Geometry: final body of the model. Coordinates: model frame, mm. Round coordinates to 2 decimals unless told otherwise and drop trailing zeros. Write each loop counter-clockwise with the first axis right and the second up, starting at its lowest first coordinate (ties: lowest second). Pieces come first, ordered by that corner, then holes. Notation, with made-up numbers: M 57.25,-6 L 92.25,-6 A11 cw 92.25,0 Z; hole C 11.5,38.25 d7. An arc over 180 degrees is marked long. Answer as CSV lines item,"result". Start each with the question number.
Q1. Section query B-B on y = -1.5. Output: boundary loops of the cut face in (x, z), and give its area (3 significant figures).
Q2. Section query C-C on z = -825. Output: boundary loops of the cut face in (x, y).
Q3. Ray query, probe 1 along Z at (x, y) = (418, 36); probe 2 along X at (y, z) = (-106, -161). Return the intervals inside material, ascending.
Q4. Section query A-A on x = -86. Output: boundary loops of the cut face in (y, z), and give its area (3 significant figures).
```python
from build123d import *

# Parameters (mm, degrees)
F0_W     = 412.1005833149
F0_H     = 230.7337969542
F1_DEPTH = 15
F2_R     = 6.4013337275
F3_DEPTH = 1000
F4_DEPTH = 1000
F5_DEPTH = 134.62


with BuildPart() as f1:
    # F0 (on Top) → F1 (new body)
    with BuildSketch(Plane.XY):
        Rectangle(F0_W, F0_H)
    extrude(amount=F1_DEPTH)

    # F2 (on face) → F3 (join)
    with BuildSketch(Plane(origin=(0, 0, 0), x_dir=(1, 0, 0), z_dir=(0, 0, -1))):
        with Locations((-190.1699453592, 101.8757298589)):
            Circle(F2_R)
    extrude(amount=F3_DEPTH)

    # F4 (add): a face of the model
    f4_faces = [f1.faces().sort_by_distance(p)[0] for p in [
        (206.0502916574, 0, 7.5),
    ]]
    extrude(f4_faces, amount=F4_DEPTH)

    # F5 (add): a face of the model
    f5_faces = [f1.faces().sort_by_distance(p)[0] for p in [
        (500, -115.3668984771, 7.5),
    ]]
    extrude(f5_faces, amount=F5_DEPTH)


solid = f1.part
```
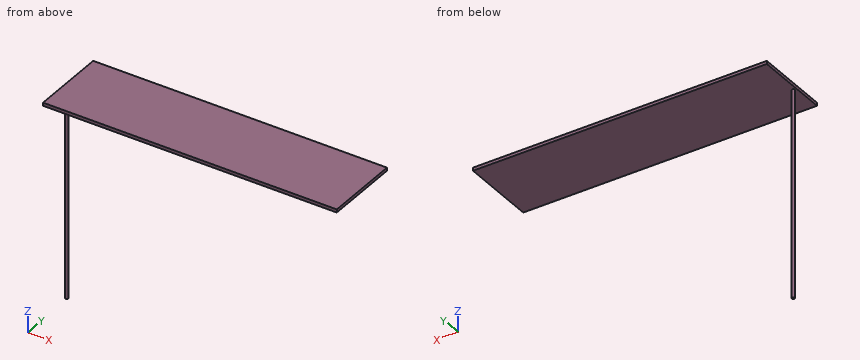
Entries:
1,outline,"M -206.05,0 L 1206.05,0 L 1206.05,15 L -206.05,15 Z"
1,area,"21,200 mm^2"
2,outline,"C -190.17,-101.88 d12.8"
3,probe 1,"z = 0 to 15"
3,probe 2,"x = -195.07 to -185.27"
4,outline,"M -249.99,0 L 115.37,0 L 115.37,15 L -249.99,15 Z"
4,area,"5,480 mm^2"
